```python
from build123d import *

# Parameters (mm, degrees)
PAD_DEPTH    = 20
SKETCH001_W  = 30
SKETCH001_H  = 8
PAD001_DEPTH = 4
SKETCH002_W  = 30
SKETCH002_H  = 8
PAD002_DEPTH = 4


with BuildPart() as part:
    # Sketch → Pad (new body)
    with BuildSketch(Plane.XY):
        Polygon((9.109291, 30.803959), (-16.390709, 5.303959), (-16.390709, 0.803959), (13.609291, 0.803959), (13.609291, 30.803959), align=None)
    extrude(amount=PAD_DEPTH)

    # Sketch001 (on Face4 of Pad) → Pad001 (join)
    with BuildSketch(Plane.YZ.offset(13.609291)):
        with Locations((15.803959, 10)):
            Rectangle(SKETCH001_W, SKETCH001_H)
    extrude(amount=PAD001_DEPTH)

    # Sketch002 (on Face9 of Pad001) → Pad002 (join)
    with BuildSketch(Plane.XZ.offset(-0.803959)):
        with Locations((-1.390709, 10)):
            Rectangle(SKETCH002_W, SKETCH002_H)
    extrude(amount=PAD002_DEPTH)


solid = part.part
```
Part model, mm, in its own coordinate system. A direction names the side the tool comes from. Coordinates: 2 decimals unless noted, no trailing zeros. Write each loop counter-clockwise with the first axis right and the second up, starting at its lowest first coordinate (ties: lowest second). Pieces come first, ordered by that corner, then holes.
Item 1: Slice it at A-A (z = 11.25). Write the cut outline in (x, y), and give its area (3 significant figures).
Item 2: Which spindle directions (+Z, -Z, +X, -X, +Y, -Y) get a long thin tool onto all of the face, cutting with end or side? Do faces 1 (the face through (-2, -1, 14)), 2 (the face through (13.609, 16, 17)), 3 (the face through (-2, -1, 6)). Say none if no direction does.
Item 3: Pin check, flat tips, straight feed: pin 1 (2 mm diameter, centred on x = -3.5, y = -2, fed in from -Z); pin 2 (12 mm diameter, centred on y = 13.5, z = 5, fed in from -X); pin 3 (1.2 mm diameter, centred on x = 16, z = 9.5, fed in from -Y); pin 4 (1 mm diameter, centred on x = -0.5, y = 22.5, fed in from +Z). Stop position of each tip, or through.
Item 4: Slice it at D-D (z = 15.75). Write the cut outline in (x, y).
Item 5: Slice it at C-C (y = 3.5). Write the cut outline in (x, z), and give its area (3 significant figures).
Item 6: Probe line 1 (Z direction, x = -8, y = 0.5); line 2 (Y direction, x = 15, z = 9); line 3 (X direction, y = 4, z = 17.25). List the from-to ranges inside material, lowest first.
Item 7: Slice it at B-B (x = 10). Write the cut outline in (y, z), and give its area (3 significant figures).
Results found:
1. outline: (-16.39, -3.2) - (13.61, -3.2) - (13.61, 0.8) - (17.61, 0.8) - (17.61, 30.8) - (9.11, 30.8) - (-16.39, 5.3) - close
1. area: 815 mm2
2. face 1: +Z, +X, -X, -Y
2. face 2: +Z, +X, +Y, -Y
2. face 3: -Z, +X, -X, -Y
3. pin 1: stops at z = 6
3. pin 2: stops at x = -14.19
3. pin 3: stops at y = 0.8
3. pin 4: passes through
4. outline: (-16.39, 0.8) - (13.61, 0.8) - (13.61, 30.8) - (9.11, 30.8) - (-16.39, 5.3) - close
5. outline: (-16.39, 0) - (13.61, 0) - (13.61, 6) - (17.61, 6) - (17.61, 14) - (13.61, 14) - (13.61, 20) - (-16.39, 20) - close
5. area: 632 mm2
6. line 1: z = 6 to 14
6. line 2: y = 0.8 to 30.8
6. line 3: x = -16.39 to 13.61
7. outline: (-3.2, 6) - (0.8, 6) - (0.8, 0) - (30.8, 0) - (30.8, 20) - (0.8, 20) - (0.8, 14) - (-3.2, 14) - close
7. area: 632 mm2
